from build123d import *

# Parameters (mm, degrees)
BOSS_EXTRUDE1_DEPTH = 2
SKETCH2_R           = 7.5
CUT_EXTRUDE1_DEPTH  = 10


with BuildPart() as part:
    # Sketch1 → Boss-Extrude1 (new body)
    with BuildSketch(Plane(origin=(0, 0, 0), x_dir=(1, 0, 0), z_dir=(0, 1, 0))):
        Polygon((-175, 55.76), (-131.59, 175), (0, 175), (0, 0), (-175, 0), align=None)
    extrude(amount=BOSS_EXTRUDE1_DEPTH)

    # Sketch2 → Cut-Extrude1 (cut)
    with BuildSketch(Plane.XZ):
        with Locations(Location((-145, -40, 0), (0, 0, 270))):
            Circle(SKETCH2_R)
    extrude(amount=-CUT_EXTRUDE1_DEPTH, mode=Mode.SUBTRACT)


solid = part.part
Geometry: final body of the model. Coordinates: model frame, mm. Give positions to 0.01 mm unless a question says otherwise; leave off trailing zeros. Write each loop counter-clockwise with the first axis right and the second up, starting at its lowest first coordinate (ties: lowest second). Pieces come first, ordered by that corner, then holes.
(1) Cut plane A-A, the plane z = -40. Return loops of the section in (x, y).
(2) First-contact query: P1, Ø9, axis at x = -145, z = -40, coming from the -Y side. Flat tip, straight axial feed; report the tip coordinate or a pass-through.
(3) Cut plane D-D, the plane z = -124. Return loops of the section in (x, y).
(4) Cut plane B-B, the plane x = -145. Return loops of the section in (y, z).
(5) Mould query, pull axis Z, two halves, no side actions, for faces 1 (the cylindrical face through (-137.564, 0.986, -39.024)), 2 (the flat face through (-153.599, 0.986, -114.545)), 3 (the flat face through (-86, 0, -89)). Classes: released by +Z, released by -Z, zero draft, split by the parting line, or undercut.
(6) Cut plane C-C, the plane y = 1.1. Return loops of the section in (x, z), then the cut area to 3 significant figures.
(7) Ray query, line 1 (X direction, y = 0.45, z = -40); line 2 (X direction, y = 0.1, z = -43); line 3 (X direction, y = 1.65, z = -124.5). Return the intervals inside material, ascending.
Values follow:
1. outline: (-175, 0) - (-152.5, 0) - (-152.5, 2) - (-175, 2) - close; (-137.5, 0) - (0, 0) - (0, 2) - (-137.5, 2) - close
2. P1: passes through
3. outline: (-150.16, 0) - (0, 0) - (0, 2) - (-150.16, 2) - close
4. outline: (0, -138.16) - (2, -138.16) - (2, -47.5) - (0, -47.5) - close; (0, -32.5) - (2, -32.5) - (2, 0) - (0, 0) - close
5. face 1: undercut
5. face 2: released by -Z
5. face 3: zero draft
6. outline: (-175, -55.76) - (-131.59, -175) - (0, -175) - (0, 0) - (-175, 0) - close; hole circle Ø15 at (-145, -40)
6. area: 27,900 mm2
7. line 1: x = -175 to -152.5, -137.5 to 0
7. line 2: x = -175 to -151.87, -138.13 to 0
7. line 3: x = -149.97 to 0
